```python
from build123d import *

# Parameters (mm, degrees)
BOSS_EXTRUDE1_DEPTH = 25
CUT_EXTRUDE1_DEPTH  = 25


with BuildPart() as part:
    # Sketch1 → Boss-Extrude1 (new body)
    with BuildSketch(Plane.XY):
        Polygon((47.177011042, 107.177011042), (-60, 0), (60, 0), (60, 120), (47.177011042, 120), align=None)
        Polygon((47.177011042, 89.789277975), (47.177011042, 11.03307526), (-29.533576018, 11.03307526), align=None, mode=Mode.SUBTRACT)
    extrude(amount=BOSS_EXTRUDE1_DEPTH)

    # Sketch2 → Cut-Extrude1 (cut)
    with BuildSketch(Plane.XY.offset(25)):
        with BuildLine():
            Line((25.294500052, 72.229110711), (-11.022426811, 35.912183847))
            ThreePointArc((-11.022426811, 35.912183847), (-15.729304171, 35.912183847), (-15.729304171, 40.619061207))
            Line((-15.729304171, 40.619061207), (20.587622692, 76.93598807))
            ThreePointArc((20.587622692, 76.93598807), (25.294500052, 76.93598807), (25.294500052, 72.229110711))
        make_face()
    extrude(amount=-CUT_EXTRUDE1_DEPTH, mode=Mode.SUBTRACT)


solid = part.part
```
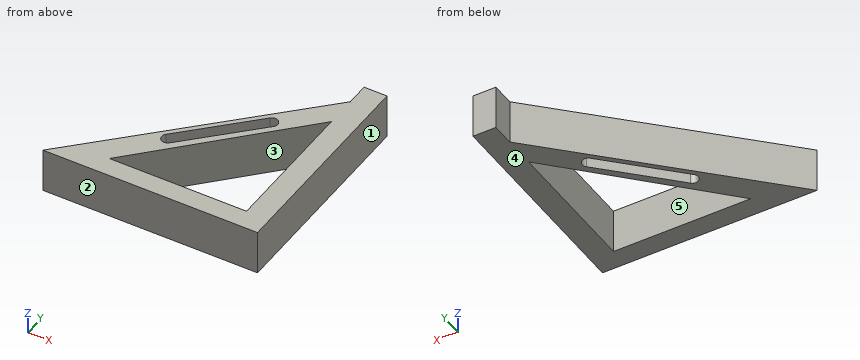
Design review of the part built by this model. Coordinates are the model's own, in mm. Face numbers are marked on the shaded views. A direction names the side the tool comes from. Round coordinates to 2 decimals unless told otherwise and drop trailing zeros. Order: outer loops, then holes, each group sorted by start corner. A loop starts at its lowest first (then second) coordinate and runs counter-clockwise, first axis right, second up. Notation, with made-up numbers: M 86,72.25 L 118,72.25 A32 ccw 118,98.25 Z; hole C 15.5,51 d5. An arc over 180 degrees is marked long. Put each result on its own line as item: value.
Q1. Insertion check: pin 1 Ø1 at (y, z) = (82.5, 4.5) entering from -X; pin 2 Ø2 at (y, z) = (66, 21) entering from -X; pin 3 Ø3 at (x, z) = (-47, 4.5) entering from +Y. Each pin has a flat end and moves straight along its axis. Give the tip position at first contact, or say it passes through.
Reported:
pin 1: x = 22
pin 2: x = 5
pin 3: y = 14.5
Q2. To check wall thickness, follow line 1 (X direction, y = 70, z = 17.25); line 2 (X direction, y = 46, z = 13.25); line 3 (Y direction, x = 18, z = 19.25). State the ranges of each line that lie inside material, in increasing order.
Reported:
line 1: 10 to 13.65, 23.07 to 27.9, 47.18 to 60
line 2: -14 to -10.35, -0.93 to 4.53, 47.18 to 60
line 3: 0 to 11.03, 59.83 to 64.93, 74.35 to 78
Q3. Consider section D-D (x = -4). State the section outline as (y, z) points, and give its area (3 significant figures).
Reported:
outline: M 0,0 L 11.03,0 L 11.03,25 L 0,25 Z; M 37.25,0 L 42.93,0 L 42.93,25 L 37.25,25 Z; M 52.35,0 L 56,0 L 56,25 L 52.35,25 Z
area: 509 mm²
Q4. Draft analysis for pull direction X (two halves, no side actions). For the marked faces 1, 2 and 3, state which applies: released by +X, released by -X, zero draft, split by the parting line, or undercut.
Reported:
face 1: released by +X
face 2: zero draft
face 3: undercut
Q5. Machinability: for the marked faces 4 and 5, which of the approach directions +Z, -Z, +X, -X, +Y, -Y give a long, thin tool a straight path to every point of the face, cutting with its end or side? Answer none if there is none.
Reported:
face 4: -Z, +X, -X, +Y, -Y
face 5: +Z, -Z
Q6. Consider section B-B (x = 45). State the section outline as (y, z) points, and give its area (3 significant figures).
Reported:
outline: M 0,0 L 11.03,0 L 11.03,25 L 0,25 Z; M 87.55,0 L 105,0 L 105,25 L 87.55,25 Z
area: 712 mm²
Q7. Consider section A-A (z = 4.25). State the section outline as (x, y) points.
Reported:
outline: M -60,0 L 60,0 L 60,120 L 47.18,120 L 47.18,107.18 Z; hole M -29.53,11.03 L 47.18,11.03 L 47.18,89.79 Z; hole M -15.73,40.62 A3.33 ccw -11.02,35.91 L 25.29,72.23 A3.33 ccw 20.59,76.94 Z
Q8. Consider section C-C (y = 58). State the section outline as (x, z) points, and give its area (3 significant figures).
Reported:
outline: M -2,0 L 1.65,0 L 1.65,25 L -2,25 Z; M 11.07,0 L 16.21,0 L 16.21,25 L 11.07,25 Z; M 47.18,0 L 60,0 L 60,25 L 47.18,25 Z
area: 541 mm²
